Read the model definition and answer for the solid it produces. Units are mm, in the model's axes. A direction names the side the tool comes from. Coordinates: 2 decimals unless noted, no trailing zeros. Write each loop counter-clockwise with the first axis right and the second up, starting at its lowest first coordinate (ties: lowest second). Pieces come first, ordered by that corner, then holes.
Item 1: Each of these flat-tipped pins is pushed along its axis until it touches: P1, Ø6, axis at x = 8.5, y = 67, coming from the +Z side; P2, Ø10, axis at x = 9, y = -125.5, coming from the +Z side. Where does it stop, or does it pass through?
Item 2: Determine the mould class of faces 4 (the face through (30.48, 48, 34)), 5 (the face through (15.03, 6.76, 65.71)), 6 (the face through (15.027, 56.169, 77.525)), 7 (the face through (15.027, -153.599, 37.956)) for opening direction Y: released by +Y, released by -Y, zero draft, split by the parting line, or undercut.
Item 3: Straight lines are drawn through the part: probe 1 along Y at (x, z) = (4.5, 29); probe 2 along Y at (x, z) = (8, 30); probe 3 along Z at (x, y) = (11, 139.5). For each, find the intervals that lie inside material, in ascending order.
Item 4: Section C-C (y = 127) is taken. Give the vertices of the cut face in (x, z), then the cut area to 3 significant figures.
Item 5: Section B-B (y = -68) is taken. Give the vertices of the cut face in (x, z), then the cut area to 3 significant figures.
Item 6: A tool of negligible diameter and unlimited length cuts with its end or side. For faces 1 (the face through (15.027, -54.785, 61.585)), 2 (the face through (15.027, 105.576, 89.34)), 3 (the face through (15.03, 36.34, 73.08)), from which of +Z, -Z, +X, -X, +Y, -Y can it reach the whole face along a straight path? Write none if from no direction.
from build123d import *

# Parameters (mm, degrees)
F1_DEPTH = 30.48
F2_R     = 19.05
F3_DEPTH = 30.48


with BuildPart() as f1:
    # F0 (on Right) → F1 (new body)
    with BuildSketch(Plane.YZ):
        Polygon((-163.618337, 35.56), (-163.618337, 0), (186.901663, 0), (186.901663, 119.38), (132.82371, 106.448315), (137.549597, 86.685512), (107.905393, 79.596681), (103.179505, 99.359484), (83.416702, 94.633596), (88.14259, 74.870793), (58.498385, 67.781962), (53.772497, 87.544765), (34.009694, 82.818877), (38.735582, 63.056074), (9.091377, 55.967242), (4.36549, 75.730045), (-15.397313, 71.004158), (-10.671426, 51.241355), (-40.31563, 44.152523), (-45.041518, 63.915326), (-64.804321, 59.189438), (-60.078433, 39.426635), (-89.722638, 32.337804), (-94.448526, 52.100607), (-114.211329, 47.374719), (-109.485441, 27.611916), (-139.129646, 20.523085), (-143.855533, 40.285888), align=None)
    extrude(amount=F1_DEPTH)

    # F2 (on face) → F3 (cut, through all)
    with BuildSketch(Plane(origin=(0, 0, 0), x_dir=(0, -1, 0), z_dir=(-1, 0, 0))):
        with Locations((-156.421663, 30.48)):
            Circle(F2_R)
    extrude(amount=-F3_DEPTH, mode=Mode.SUBTRACT)


solid = f1.part
Established:
1. P1: stops at z = 70.53
1. P2: stops at z = 24.98
2. face 4: zero draft
2. face 5: undercut
2. face 6: undercut
2. face 7: released by -Y
3. probe 1: y = -163.62 to -141.16, -109.82 to 137.43, 175.41 to 186.9
3. probe 2: y = -163.62 to -141.4, -110.06 to 137.38, 175.47 to 186.9
3. probe 3: z = 0 to 21.73, 39.23 to 108.04
4. outline: (0, 0) - (30.48, 0) - (30.48, 84.16) - (0, 84.16) - close
4. area: 2,570 mm2
5. outline: (0, 0) - (30.48, 0) - (30.48, 37.53) - (0, 37.53) - close
5. area: 1,140 mm2
6. face 1: +Z, +X, -X, -Y
6. face 2: +Z, +X, -X
6. face 3: +X, -X
